Geometry: final body of the model. Coordinates: model frame, mm. Face numbers are marked on the shaded views. A direction names the side the tool comes from. Give positions to 0.01 mm unless a question says otherwise; leave off trailing zeros. Order: outer loops, then holes, each group sorted by start corner. A loop starts at its lowest first (then second) coordinate and runs counter-clockwise, first axis right, second up. Notation, with made-up numbers: (8.5, 86.5) -> (15.5, 86.5) arc R15 ccw to (15.5, 97.5) -> close; hole circle Ø4 at (50, 21.25). An arc over 180 degrees is marked (long way). Answer in a Markdown table with one row per item. Add a question column.
Q1. Line query: line 1 along Z through (x, y) = (12, 8.25); line 2 along X through (y, z) = (8.5, 24); line 3 along X through (y, z) = (19.25, 22.5). Output: solid intervals per line, ascending. Write a range as from..to.
Q2. Cut plane D-D on y = 9. Return the cut outline in (x, z), and give its area (3 significant figures).
Q3. Pull-direction query (X, two-part tool) for the marked faces 4, 5, 6 and 7; classes: +X half, -X half, draft (parallel to the pull), parting line (faces both ways), or undercut.
Q4. Set-up query: the marked faces 1, 2 and 3. Return all of +Z, -Z, +X, -X, +Y, -Y with unobstructed straight access to the full face (end or side cutting, diameter ignored); none if empty.
Q5. Cut plane C-C on x = -12. Return the cut outline in (y, z), and give its area (3 significant figures).
Q6. Cut plane A-A on z = 24. Return the cut outline in (x, y), and give its area (3 significant figures).
Q7. Contact query for flat-ended pins moving along their axis: P1, Ø8, axis at y = 3, z = 5.5, coming from the -X side; P2, Ø9, axis at x = 0.5, z = 10, coming from the +Y side; P3, Ø3, axis at x = 12, z = 24, coming from the -Y side; P4, Ø3, axis at x = -12, z = 4.5, coming from the -Y side. Output: stop coordinate, or through.
Q8. Cut plane B-B on x = 0. Return the cut outline in (y, z).
from build123d import *

# Parameters (mm, degrees)
BOSS_EXTRUDE1_OUTLINE_R = 4
BOSS_EXTRUDE1_DEPTH     = 30
CUT_EXTRUDE1_DEPTH      = 41.902322672
CUT_EXTRUDE1_DEPTH_BACK = 41.902322672
SKETCH2_R               = 1.7


# Read off the part's stored shape, not the designer's step: Boss-Extrude1
with BuildPart() as part:
    # Boss-Extrude1 outline → Boss-Extrude1 (new body)
    with BuildSketch(Plane.XY):
        Polygon((7, 0), (11, 4), (15, 4), (15, 14), (17, 16), (17, 21), (16, 22), (10, 22), (9, 21), (-9, 21), (-10, 22), (-16, 22), (-17, 21), (-17, 16), (-15, 14), (-15, 4), (-11, 4), (-7, 0), align=None)
        with Locations((0, 11)):
            Circle(BOSS_EXTRUDE1_OUTLINE_R, mode=Mode.SUBTRACT)
    extrude(amount=BOSS_EXTRUDE1_DEPTH)

    # Sketch2 → Cut-Extrude1 (cut, two sides: drawn at the far end of the back side and taken through both)
    with BuildSketch(Plane(origin=(0, 22, 0), x_dir=(1, 0, 0), z_dir=(0, 1, 0)).offset(-CUT_EXTRUDE1_DEPTH_BACK)):
        with Locations(Location((12, -6, 0), (0, 0, 233.968120928))):
            Circle(SKETCH2_R)
        with Locations(Location((-12, -6, 0), (0, 0, 53.968120928))):
            Circle(SKETCH2_R)
        with Locations(Location((12, -24, 0), (0, 0, 126.031879072))):
            Circle(SKETCH2_R)
        with Locations(Location((-12, -24, 0), (0, 0, 306.031879072))):
            Circle(SKETCH2_R)
    extrude(amount=CUT_EXTRUDE1_DEPTH + CUT_EXTRUDE1_DEPTH_BACK, mode=Mode.SUBTRACT)


solid = part.part
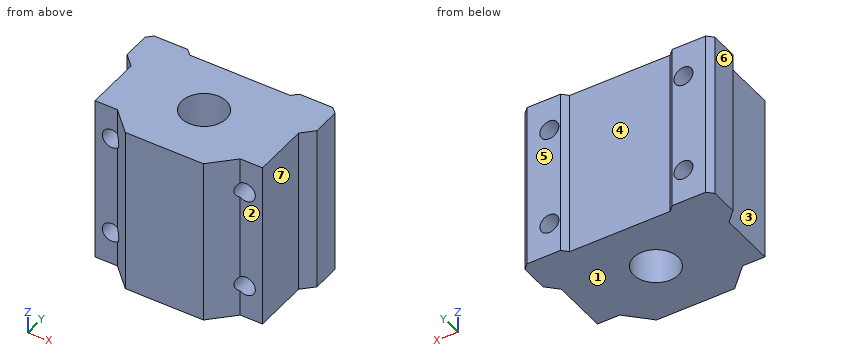
Completed:
| question | item | result |
|---|---|---|
| 1 | line 1 | z = 0..4.3, 7.7..22.3, 25.7..30 |
| 1 | line 2 | x = -15..-13.7, -10.3..-3.12, 3.12..10.3, 13.7..15 |
| 1 | line 3 | x = -17..-12.8, -11.2..11.2, 12.8..17 |
| 2 | outline | (-15, 0) -> (-3.46, 0) -> (-3.46, 30) -> (-15, 30) -> close; (3.46, 0) -> (15, 0) -> (15, 30) -> (3.46, 30) -> close; hole circle Ø3.4 at (-12, 6); hole circle Ø3.4 at (-12, 24); hole circle Ø3.4 at (12, 6); hole circle Ø3.4 at (12, 24) |
| 2 | area | 656 mm² |
| 3 | face 4 | undercut |
| 3 | face 5 | draft |
| 3 | face 6 | -X half |
| 3 | face 7 | +X half |
| 4 | face 1 | -Z, +X, -X, +Y, -Y |
| 4 | face 2 | +Z, -Z, +X, -Y |
| 4 | face 3 | +Z, -Z, -X, -Y |
| 5 | outline | (4, 0) -> (22, 0) -> (22, 4.3) -> (4, 4.3) -> close; (4, 7.7) -> (22, 7.7) -> (22, 22.3) -> (4, 22.3) -> close; (4, 25.7) -> (22, 25.7) -> (22, 30) -> (4, 30) -> close |
| 5 | area | 418 mm² |
| 6 | outline | (-17, 16) -> (-15, 14) -> (-15, 4) -> (-13.7, 4) -> (-13.7, 22) -> (-16, 22) -> (-17, 21) -> close; (-10.3, 3.3) -> (-7, 0) -> (7, 0) -> (10.3, 3.3) -> (10.3, 22) -> (10, 22) -> (9, 21) -> (-9, 21) -> (-10, 22) -> (-10.3, 22) -> close; (13.7, 4) -> (15, 4) -> (15, 14) -> (17, 16) -> (17, 21) -> (16, 22) -> (13.7, 22) -> close; hole circle Ø8 at (0, 11) |
| 6 | area | 447 mm² |
| 7 | P1 | stops at x = -15 |
| 7 | P2 | stops at y = 21 |
| 7 | P3 | passes through |
| 7 | P4 | stops at y = 3.5 |
| 8 | outline | (0, 0) -> (7, 0) -> (7, 30) -> (0, 30) -> close; (15, 0) -> (21, 0) -> (21, 30) -> (15, 30) -> close |
